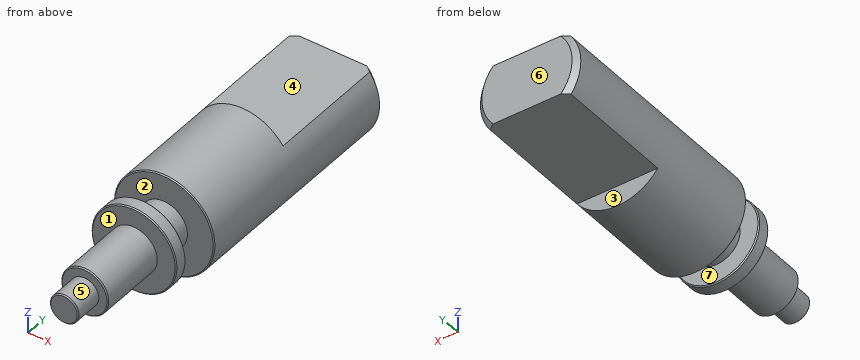
```python
from build123d import *

# Parameters (mm, degrees)
CUT_EXTRUDE_1_DEPTH = 6.15
CHAMFER_1_SIZE      = 0.25
CHAMFER_2_SIZE      = 0.05


with BuildPart() as part:
    # Эскиз1 → Повернуть1 (revolve)
    with BuildSketch(Plane.XY):
        Polygon((0, 18.3), (0, 0), (-0.7, 0), (-0.7, 1.4), (-1.15, 1.4), (-1.15, 4.75), (-2.075, 4.75), (-2.075, 5.4), (-1.15, 5.4), (-1.15, 6.8), (-2.46, 6.8), (-2.46, 18.3), align=None)
    revolve(axis=Axis((0, 18.3, 0), (0, -1, 0)))

    # Эскиз2 → Вырез-Вытянуть1 (cut)
    with BuildSketch(Plane(origin=(0, 18.3, 0), x_dir=(1, 0, 0), z_dir=(0, 1, 0))):
        with BuildLine():
            Line((-1.979898987, 1.46), (1.979898987, 1.46))
            ThreePointArc((1.979898987, 1.46), (0, 2.46), (-1.979898987, 1.46))
        make_face()
        with BuildLine():
            Line((-1.979898987, -1.46), (1.979898987, -1.46))
            ThreePointArc((1.979898987, -1.46), (0, -2.46), (-1.979898987, -1.46))
        make_face()
    extrude(amount=-CUT_EXTRUDE_1_DEPTH, mode=Mode.SUBTRACT)

    # Фаска1
    chamfer_1_edges = [part.edges().sort_by_distance(p)[0] for p in [
        (-2.336894468, 18.3, -0.768455754),
        (2.46, 18.3, 0),
    ]]
    chamfer(chamfer_1_edges, length=CHAMFER_1_SIZE)

    # Фаска2
    chamfer_2_edges = [part.edges().sort_by_distance(p)[0] for p in [
        (2.075, 5.4, 0),
        (2.075, 4.75, 0),
        (1.15, 1.4, 0),
        (0.7, 0, 0),
        (2.46, 6.8, 0),
    ]]
    chamfer(chamfer_2_edges, length=CHAMFER_2_SIZE)


solid = part.part
```
The model under review builds one solid part; all positions refer to its coordinate system, in mm. Face numbers are marked on the shaded views. A direction names the side the tool comes from. Coordinates: 2 decimals unless noted, no trailing zeros. Loops run counter-clockwise (first coordinate to the right, second up) from the corner with the lowest first, then second, coordinate; pieces in that order, holes last. Notation, with made-up numbers: (9, 86.25) -> (28, 86.25) arc R26 ccw to (28, 101.25) -> close; hole circle Ø6 at (69, 51). An arc over 180 degrees is marked (long way). Answer as CSV lines item,"result".
Item 1: Take a section at C-C, the plane y = 16. State the section outline as (x, z) points.
Results below:
outline,"(-1.98, -1.46) -> (1.98, -1.46) arc R2.46 ccw to (1.98, 1.46) -> (-1.98, 1.46) arc R2.46 ccw to start"
Item 2: Take a section at D-D, the plane y = 4.5. State the section outline as (x, z) points.
Results below:
outline,"circle Ø2.3 at (0, 0)"
Item 3: Machinability: for the marked faces 1, 2, 3 and 4, which of the approach directions +Z, -Z, +X, -X, +Y, -Y give a long, thin tool a straight path to every point of the face, cutting with its end or side? Answer none if there is none.
Results below:
face 1,"-Y"
face 2,"none"
face 3,"-Z, +X, -X, +Y"
face 4,"+Z, +X, -X, +Y"
Item 4: For L1, parallel to Y at x = -0.55, z = 1.35; L2, parallel to Z at x = 1.5, y = 14; L3, parallel to Y at x = 0.8, z = -0.4, list the stretches that pass through material, from the lowest coordinate up.
Results below:
L1,"y = 4.75 to 5.4, 6.8 to 18.3"
L2,"z = -1.46 to 1.46"
L3,"y = 1.4 to 18.3"
Item 5: Draft analysis for pull direction Y (two halves, no side actions). For the marked faces 5, 6 and 7, state which applies: +Y half, -Y half, draft (parallel to the pull), parting line (faces both ways), or undercut.
Results below:
face 5,"draft"
face 6,"+Y half"
face 7,"undercut"
Item 6: Insertion check: pin 1 (0.5 mm diameter, centred on x = 0, z = 2, fed in from +Y); pin 2 (1 mm diameter, centred on x = -1.5, y = 6.5, fed in from -Z); pin 3 (1.5 mm diameter, centred on x = -0.5, y = 6, fed in from +Z). Each pin has a flat end and moves straight along its axis. Give the tip position at first contact, or say it passes through.
Results below:
pin 1,"stops at y = 12.15"
pin 2,"stops at z = -2.18"
pin 3,"stops at z = 2.07"
